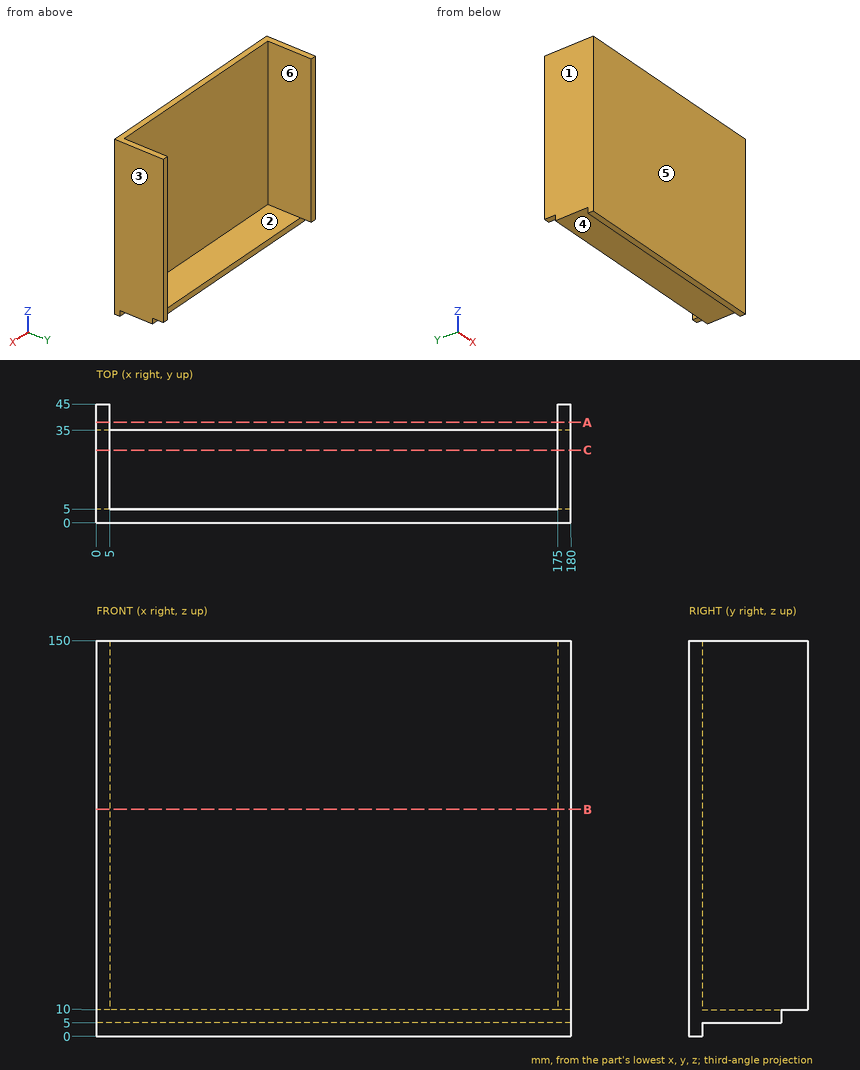
Could you check a few things on this drawing? It's one solid part, dimensions in mm from its lowest x, y, z. A direction names the side the tool comes from. Give positions to 0.01 mm unless a question says otherwise; leave off trailing zeros. Write each loop counter-clockwise with the first axis right and the second up, starting at its lowest first coordinate (ties: lowest second). Pieces come first, ordered by that corner, then holes.
(1) Will these pins go through, and if not, where does the flat tip stop? pin 1 (12 mm diameter, centred on x = 19.5, y = 20, fed in from +Z); pin 2 (12 mm diameter, centred on x = 35, z = 39.5, fed in from +Y); pin 3 (15 mm diameter, centred on x = 124.5, y = 23, fed in from -Z).
Output values:
pin 1: stops at z = 10
pin 2: stops at y = 5
pin 3: stops at z = 5
(2) Imagine slicing it at B-B, the plane z = 86. Write out the boundary of the cut face in (x, y).
Output values:
outline: (0, 0) - (180, 0) - (180, 45) - (175, 45) - (175, 5) - (5, 5) - (5, 45) - (0, 45) - close
(3) Thinking about a two-plate mould opening in X: for the marked faces 1, 2 and 3, which applies, pulls with the +X half, pulls with the -X half, needs draft (parallel to the pull), parting line crosses it, or undercut?
Output values:
face 1: pulls with the -X half
face 2: undercut
face 3: pulls with the +X half
(4) Imagine slicing it at A-A, the plane y = 38. Write out the boundary of the cut face in (x, z).
Output values:
outline: (0, 10) - (5, 10) - (5, 150) - (0, 150) - close; (175, 10) - (180, 10) - (180, 150) - (175, 150) - close
(5) On a 3-axis mill with a long thin cutter (end or side, diameter ignored), from which of +Z, -Z, +X, -X, +Y, -Y can I reach the whole of each face in a straight line? I mean the marked faces 4, 5 and 6. Say none if no direction works.
Output values:
face 4: -Z, +X, -X, +Y
face 5: +Z, -Z, +X, -X, -Y
face 6: +Z, +Y
(6) If I drill on L1, parallel to X at y = 8, z = 52; L2, parallel to Y at x = 111.5, z = 93; L3, parallel to Z at x = 169.5, y = 27, over which ranges is the centre line in solid material (lowest first)?
Output values:
L1: x = 0 to 5, 175 to 180
L2: y = 0 to 5
L3: z = 5 to 10
(7) Imagine slicing it at C-C, the plane y = 27.5. Write out the boundary of the cut face in (x, z), and give its area (3 significant figures).
Output values:
outline: (0, 5) - (180, 5) - (180, 150) - (175, 150) - (175, 10) - (5, 10) - (5, 150) - (0, 150) - close
area: 2,300 mm2
